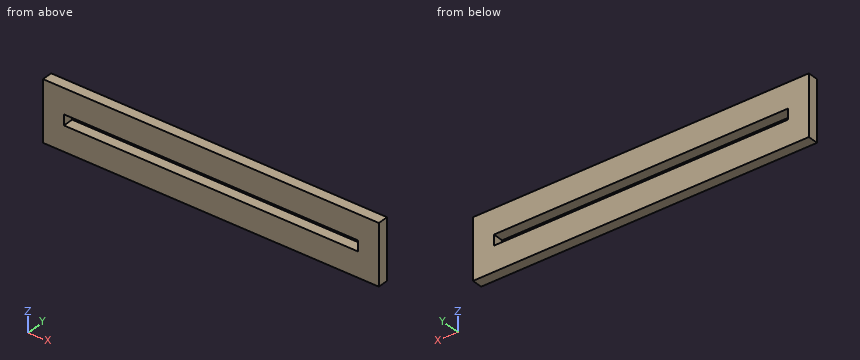
```python
from build123d import *

# Parameters (mm, degrees)
F0_W     = 112
F0_H     = 4
F1_DEPTH = 4


with BuildPart() as f1:
    # F0 (on Front) → F1 (new body)
    with BuildSketch(Plane.XZ):
        Polygon((128, 0), (0, 0), (0, -23), (128, -23), (128, -13.5), (128, -11.5), (128, -9.5), align=None)
        with Locations((64, -11.5)):
            Rectangle(F0_W, F0_H, mode=Mode.SUBTRACT)
    extrude(amount=F1_DEPTH)


solid = f1.part
```
Can you work these out from the model? Positions are in its coordinate system, mm. Give positions to 0.01 mm unless a question says otherwise; leave off trailing zeros. Order: outer loops, then holes, each group sorted by start corner. A loop starts at its lowest first (then second) coordinate and runs counter-clockwise, first axis right, second up. Notation, with made-up numbers: M 24,-16.75 L 76,-16.75 A17 ccw 76,-8.75 Z; hole C 28.25,4.25 d11. An arc over 180 degrees is marked long. One line per item, written item: value.
1) For P1, Ø1, axis at y = -1, z = -12.5, coming from the -X side, with a flat end and sliding along its axis, tell me the tip position at first contact or that it passes through.
Answer sheet:
P1: stops at x = 0
2) I want a section at C-C, the plane y = -1.4. List the corners of the cut face in (x, z) for me.
Answer sheet:
outline: M 0,-23 L 128,-23 L 128,0 L 0,0 Z; hole M 8,-13.5 L 120,-13.5 L 120,-9.5 L 8,-9.5 Z
3) I want a section at B-B, the plane z = -12. List the corners of the cut face in (x, y) for me.
Answer sheet:
outline: M 0,-4 L 8,-4 L 8,0 L 0,0 Z; M 120,-4 L 128,-4 L 128,0 L 120,0 Z
4) I want a section at A-A, the plane x = 116. List the corners of the cut face in (y, z) for me, plus the area to 3 significant figures.
Answer sheet:
outline: M -4,-23 L 0,-23 L 0,-13.5 L -4,-13.5 Z; M -4,-9.5 L 0,-9.5 L 0,0 L -4,0 Z
area: 76.0 mm^2
5) Please list where these lines run through material, in increasing order: line 1 along Z through (x, y) = (112.5, -3.4); line 2 along X through (y, z) = (-0.55, -12).
Answer sheet:
line 1: z = -23 to -13.5, -9.5 to 0
line 2: x = 0 to 8, 120 to 128
